Geometry: final body of the model. Coordinates: model frame, mm. A direction names the side the tool comes from. Coordinates: 2 decimals unless noted, no trailing zeros. Order: outer loops, then holes, each group sorted by start corner. A loop starts at its lowest first (then second) coordinate and runs counter-clockwise, first axis right, second up. Notation, with made-up numbers: M 71,-3.5 L 114,-3.5 A18 cw 114,26.5 Z; hole C 86.25,3 d3. An arc over 180 degrees is marked long. Use CSV: the item, a comma, the result in double quotes. Start each with the question number.
1. Section query A-A on y = 85.5. Return the cut outline in (x, z), and give its area (3 significant figures).
2. Pull-direction query (Y, two-part tool) for faces 1 (the flat face through (104, 70, 30)), 2 (the flat face through (178, 55.9, 68.2)); classes: pulls with the +Y half, pulls with the -Y half, needs draft (parallel to the pull), parting line crosses it, or undercut.
3. Section query B-B on z = 50. Return the cut outline in (x, y).
4. Material intervals for line 1 (X direction, y = 0, z = 30); line 2 (Y direction, x = -1.5, z = 32.5) (3 decimals); line 3 (Z direction, x = -52.5, y = -83), sorted ascending.
5. Section query C-C on y = 54. Return the cut outline in (x, z), and give its area (3 significant figures).
6. First-contact query: P1, Ø5, axis at y = -42, z = 28, coming from the -X side; P2, Ø4, axis at x = 132, y = 86, coming from the -Z side; P3, Ø12.5, axis at y = 52.5, z = 30.5, coming from the +X side. Flat tips, straight axial feed; report the tip coordinate or a pass-through.
7. Set-up query: faces 3 (the flat face through (98.832, 65, 20)), 4 (the flat face through (-1, -1, 40)), 5 (the flat face through (34.5, 69.8, 71.3)). Return all of +Z, -Z, +X, -X, +Y, -Y with unobstructed straight access to the full face (end or side cutting, diameter ignored); none if empty.
8. Section query D-D on z = 18. Return the cut outline in (x, y).
from build123d import *
from build123d import SkipClean  # not in build123d's __all__

# Parameters (mm, degrees)
F1_DEPTH = 46
F3_DEPTH = 74
F4_DEPTH = 143.5
F5_R     = 75
F5_R_2   = 72
F6_DEPTH = 40
F7_R     = 72
F8_DEPTH = 1


# Not quite as in the source:
# - after a boolean that leaves OpenCascade's solid faulty, fix() repairs it


with BuildPart() as f1:
    # F0 (on Top) → F1 (new body)
    with BuildSketch(Plane.XY):
        with BuildLine():
            Line((178, 107.5), (0, 107.5))
            ThreePointArc((0, 107.5), (-65.1632565178, -85.4985379992), (103.6532681588, 28.5))
            Line((103.6532681588, 28.5), (178, 28.5))
            Line((178, 28.5), (178, 107.5))
        make_face()
    extrude(amount=F1_DEPTH)

    # F2 (on face) → F3 (cut)
    with BuildSketch(Plane.YZ.offset(178)):
        with BuildLine():
            ThreePointArc((70, 0), (40.6316496888, 14.1815523673), (33.4760352645, 46))
            Line((33.4760352645, 46), (28.5, 46))
            Line((28.5, 46), (28.5, 0))
            Line((28.5, 0), (70, 0))
        make_face()
        with BuildLine():
            Line((107.5, 0), (107.5, 37.5))
            ThreePointArc((107.5, 37.5), (96.5165042945, 10.9834957055), (70, 0))
            Line((70, 0), (107.5, 0))
        make_face()
        with BuildLine():
            ThreePointArc((37.596296508, 46), (65.714796795, 4.275204538), (103.5, 37.5))
            ThreePointArc((103.5, 37.5), (103.224795462, 41.785203205), (102.403703492, 46))
            Line((102.403703492, 46), (37.596296508, 46))
        make_face()
    extrude(amount=-F3_DEPTH, mode=Mode.SUBTRACT)

    # F2 (on face) → F4 (join)
    with BuildSketch(Plane.YZ.offset(178)):
        with BuildLine():
            ThreePointArc((37.596296508, 46), (70, 71), (102.403703492, 46))
            Line((102.403703492, 46), (106.5239647355, 46))
            ThreePointArc((106.5239647355, 46), (70, 75), (33.4760352645, 46))
            Line((33.4760352645, 46), (37.596296508, 46))
        make_face()
    with SkipClean():  # cleaning this boolean's faces spoils the solid; the shape is the same uncleaned
        extrude(amount=-F4_DEPTH)

    # F5 (on face) → F6 (cut)
    with BuildSketch(Plane(origin=(0, 0, 0), x_dir=(1, 0, 0), z_dir=(0, 0, -1))):
        with BuildLine():
            ThreePointArc((98.8321859189, -27.1744186047), (-62.1324073774, 81.5218618132), (0, -102.5))
            Line((0, -102.5), (98.8321859189, -102.5))
            Line((98.8321859189, -102.5), (98.8321859189, -27.1744186047))
        make_face()
        Circle(F5_R, mode=Mode.SUBTRACT)
        Circle(F5_R_2)
    extrude(amount=-F6_DEPTH, mode=Mode.SUBTRACT)

    add(f1.part.fix(), mode=Mode.REPLACE)

    # F7 (on face) → F8 (join)
    with BuildSketch(Plane(origin=(0, 0, 0), x_dir=(1, 0, 0), z_dir=(0, 0, -1))):
        with BuildLine():
            ThreePointArc((103.6532681588, -28.5), (-65.1632565178, 85.4985379992), (0, -107.5))
            Line((0, -107.5), (104, -107.5))
            Line((104, -107.5), (104, -70))
            Line((104, -70), (104, -28.5))
            Line((104, -28.5), (103.6532681588, -28.5))
        make_face()
        with BuildLine():
            ThreePointArc((0, -102.5), (-62.1324073774, 81.5218618132), (98.8321859189, -27.1744186047))
            Line((98.8321859189, -27.1744186047), (98.8321859189, -102.5))
            Line((98.8321859189, -102.5), (0, -102.5))
        make_face(mode=Mode.SUBTRACT)
        with BuildLine():
            Line((98.8321859189, -102.5), (98.8321859189, -27.1744186047))
            ThreePointArc((98.8321859189, -27.1744186047), (-62.1324073774, 81.5218618132), (0, -102.5))
            Line((0, -102.5), (98.8321859189, -102.5))
        make_face()
        Circle(F7_R, mode=Mode.SUBTRACT)
    extrude(amount=F8_DEPTH)


solid = f1.part
Results list:
1,outline,"M -65.16,-1 L 104,-1 L 104,3.35 L 178,3.35 L 178,7.8 L 104,7.8 L 104,46 L -65.16,46 Z; M 34.5,67.2 L 178,67.2 L 178,71.65 L 34.5,71.65 Z; hole M -56.53,0 L 98.83,0 L 98.83,40 L -56.53,40 Z"
1,area,"2,700 mm²"
2,face 1,"undercut"
2,face 2,"needs draft"
3,outline,"M 34.5,34.64 L 178,34.64 L 178,38.92 L 34.5,38.92 Z; M 34.5,101.08 L 178,101.08 L 178,105.36 L 34.5,105.36 Z"
4,line 1,"x = -107.5 to -102.5, -75 to -72, 72 to 75, 102.5 to 107.5"
4,line 2,"y = -107.49 to -102.489, -74.985 to -71.984, 71.984 to 74.985, 102.489 to 107.49"
4,line 3,"z = -1 to 0, 40 to 46"
5,outline,"M -92.95,-1 L -47.62,-1 L -47.62,40 L 47.62,40 L 47.62,-1 L 104,-1 L 104,3.58 L 178,3.58 L 178,8.07 L 104,8.07 L 104,46 L -92.95,46 Z; M 34.5,66.93 L 178,66.93 L 178,71.42 L 34.5,71.42 Z; hole M -87.12,0 L -52.05,0 L -52.05,40 L -87.12,40 Z; hole M 52.05,0 L 98.83,0 L 98.83,40 L 52.05,40 Z"
5,area,"3,050 mm²"
6,P1,"stops at x = -99.98"
6,P2,"stops at z = 2.71"
6,P3,"stops at x = 104"
7,face 3,"none"
7,face 4,"-Z"
7,face 5,"+Z, -X, +Y, -Y"
8,outline,"C 0,0 d150; M 0,107.5 A107.5 ccw long 103.65,28.5 L 104,28.5 L 104,37.97 L 178,37.97 L 178,42.76 L 104,42.76 L 104,97.24 L 178,97.24 L 178,102.03 L 104,102.03 L 104,107.5 Z; hole C 0,0 d144; hole M 0,102.5 A102.5 ccw long 98.83,27.17 L 98.83,102.5 Z"
